Could you check a few things on this model? Use its own coordinates, in mm. Coordinates: 2 decimals unless noted, no trailing zeros. Order: outer loops, then holes, each group sorted by start corner. A loop starts at its lowest first (then second) coordinate and runs counter-clockwise, first axis right, second up. Notation, with made-up numbers: (-34, 50) - (0, 50) arc R23 cw to (0, 84) - close; hole circle Ø5 at (26, 7). An arc over 180 degrees is marked (long way). Answer as a JSON object with one key per item and string values. Group by question number.
(1) Imagine slicing it at C-C, the plane z = 5.1. Give the number of separate pieces and of enclosed holes in the cut face, and give its area (3 significant figures).
(2) Imagine slicing it at A-A, the plane y = 128. Write out the boundary of the cut face in (x, z), and give its area (3 significant figures).
(3) Please list where these lines run through material, in increasing order: probe 1 along Y at (x, z) = (-3, 5.35); probe 2 along X at (y, z) = (-19, 2.8); probe 3 along X at (y, z) = (-8, 3).
(4) We'd pull the mould along Z, two halves only. Please class faces 1 (the flat face through (-5, 5, 6)), 2 (the flat face through (-5, 5, 0)), 3 (the cylindrical face through (-257.96, 236.55, 2.96)): pulls with the +Z half, pulls with the -Z half, needs draft (parallel to the pull), parting line crosses it, or undercut.
(5) Will these pins go through, and if not, where does the flat tip stop? P1, Ø9, axis at x = -15.75, y = 314.55, coming from the -Z side; P2, Ø2, axis at x = 220, z = 5.5, coming from the -Y side; P3, Ø3, axis at x = 303, z = 3.5, coming from the +Y side; P4, Ø3, axis at y = 220.5, z = 3, coming from the -X side.
(6) Imagine slicing it at B-B, the plane x = 110.5. Write out the boundary of the cut face in (y, z), and give its area (3 significant figures).
from build123d import *

# Parameters (mm, degrees)
SKETCH1_R           = 350
SKETCH1_R_2         = 3.853599608
BOSS_EXTRUDE1_DEPTH = 6
SKETCH3_R           = 5
CUT_EXTRUDE1_DEPTH  = 23


with BuildPart() as part:
    # Sketch1 → Boss-Extrude1 (new body)
    with BuildSketch(Plane.XY):
        Circle(SKETCH1_R)
        with Locations((-15.75089486, 314.549698435)):
            Circle(SKETCH1_R_2, mode=Mode.SUBTRACT)
        with Locations((15.650361768, 314.54857996)):
            Circle(SKETCH1_R_2, mode=Mode.SUBTRACT)
        with Locations((0.100305228, 247.936525061)):
            Circle(SKETCH1_R_2, mode=Mode.SUBTRACT)
        with Locations((-314.54747334, -15.780069307)):
            Circle(SKETCH1_R_2, mode=Mode.SUBTRACT)
        with Locations((-314.546354865, 15.621187321)):
            Circle(SKETCH1_R_2, mode=Mode.SUBTRACT)
        with Locations((-247.934299965, 0.071130781)):
            Circle(SKETCH1_R_2, mode=Mode.SUBTRACT)
        with Locations(Location((247.926914103, 0.099183743, 0), (0, 0, 180))):
            Circle(SKETCH1_R_2, mode=Mode.SUBTRACT)
        with Locations(Location((314.538969003, 15.649240284, 0), (0, 0, 180))):
            Circle(SKETCH1_R_2, mode=Mode.SUBTRACT)
        with Locations(Location((314.540087478, -15.752016345, 0), (0, 0, 180))):
            Circle(SKETCH1_R_2, mode=Mode.SUBTRACT)
        Polygon((9.000621865, 306.449460756), (9.000621865, 293.529460756), (6.460621865, 290.989460756), (-6.459378135, 290.989460756), (-8.999378135, 293.529460756), (-8.999378135, 306.449460756), (-6.459378135, 308.989460756), (6.460621865, 308.989460756), align=None, mode=Mode.SUBTRACT)
        Polygon((-306.44723566, 8.971447418), (-293.52723566, 8.971447418), (-290.98723566, 6.431447418), (-290.98723566, -6.488552582), (-293.52723566, -9.028552582), (-306.44723566, -9.028552582), (-308.98723566, -6.488552582), (-308.98723566, 6.431447418), align=None, mode=Mode.SUBTRACT)
        Polygon((308.979849798, 6.459500381), (306.439849798, 8.999500381), (293.519849798, 8.999500381), (290.979849798, 6.459500381), (290.979849798, -6.460499619), (293.519849798, -9.000499619), (306.439849798, -9.000499619), (308.979849798, -6.460499619), align=None, mode=Mode.SUBTRACT)
    extrude(amount=BOSS_EXTRUDE1_DEPTH)

    # Sketch3 → Cut-Extrude1 (cut)
    with BuildSketch(Plane.XY.offset(6)):
        Circle(SKETCH3_R)
    extrude(amount=-CUT_EXTRUDE1_DEPTH, mode=Mode.SUBTRACT)


solid = part.part
Result set:
{
 "1": {"separate pieces": "1", "enclosed holes": "13", "area": "383,000 mm^2"},
 "2": {"outline": "(-325.75, 0) - (325.75, 0) - (325.75, 6) - (-325.75, 6) - close", "area": "3,910 mm^2"},
 "3": {"probe 1": "y = -349.99 to -4, 4 to 245.65, 250.23 to 290.99, 308.99 to 349.99", "probe 2": "x = -349.48 to -316.66, -312.43 to 312.47, 316.61 to 349.48", "probe 3": "x = -349.91 to -307.48, -292.5 to 292.52, 307.44 to 349.91"},
 "4": {"face 1": "pulls with the +Z half", "face 2": "pulls with the -Z half", "face 3": "needs draft"},
 "5": {"P1": "stops at z = 0", "P2": "stops at y = -273.02", "P3": "stops at y = 177.76", "P4": "stops at x = -273.02"},
 "6": {"outline": "(-332.1, 0) - (332.1, 0) - (332.1, 6) - (-332.1, 6) - close", "area": "3,990 mm^2"}
}
